from build123d import *

# Parameters (mm, degrees)
BOSS_EXTRUDE1_DEPTH = 20
BOSS_EXTRUDE2_DEPTH = 80
BOSS_EXTRUDE6_DEPTH = 30
BOSS_EXTRUDE7_DEPTH = 75
CUT_EXTRUDE1_REACH  = 158.605


with BuildPart() as part:
    # Sketch1 → Boss-Extrude1 (new body)
    with BuildSketch(Plane(origin=(0, 0, 0), x_dir=(1, 0, 0), z_dir=(0, 1, 0))):
        Polygon((35, 75), (0, 75), (0, 0), (65, 0), (65, 95), (35, 95), align=None)
    extrude(amount=BOSS_EXTRUDE1_DEPTH)

    # Sketch1<3> → Boss-Extrude2 (add)
    with BuildSketch(Plane(origin=(0, 0, 0), x_dir=(1, 0, 0), z_dir=(0, 1, 0))):
        Polygon((15, 130), (15, 100), (0, 100), (0, 75), (35, 75), (35, 95), (65, 95), (65, 100), (65, 130), align=None)
    extrude(amount=BOSS_EXTRUDE2_DEPTH)

    # Sketch8 → Boss-Extrude6 (add)
    with BuildSketch(Plane(origin=(65, 0, 0), x_dir=(0, 0, -1), z_dir=(1, 0, 0))):
        Polygon((95, 57.913643311), (50, 57.913643311), (0, 20), (95, 20), align=None)
    extrude(amount=-BOSS_EXTRUDE6_DEPTH)

    # Sketch9 → Boss-Extrude7 (add)
    with BuildSketch(Plane.XY.offset(-75)):
        Polygon((0, 20), (35, 57.913643311), (35, 20), align=None)
    extrude(amount=BOSS_EXTRUDE7_DEPTH)

    # Sketch10 → Cut-Extrude1 (cut, up to next)
    with BuildSketch(Plane(origin=(35, 0, 0), x_dir=(0, 0, -1), z_dir=(1, 0, 0)), mode=Mode.PRIVATE) as cut_extrude1_sk1:
        Polygon((0, 57.913643311), (50, 57.913643311), (0, 20), align=None)
    cut_extrude1_tool1 = extrude(cut_extrude1_sk1.sketch, amount=-CUT_EXTRUDE1_REACH, mode=Mode.PRIVATE) & part.part
    add(cut_extrude1_tool1.solids().sort_by_distance((35, 45.275762, -16.666667))[0], mode=Mode.SUBTRACT)


solid = part.part
Verification items for the finished model (mm, model axes). A direction names the side the tool comes from. Coordinates: 2 decimals unless noted, no trailing zeros. Loops run counter-clockwise (first coordinate to the right, second up) from the corner with the lowest first, then second, coordinate; pieces in that order, holes last. Notation, with made-up numbers: (-21, 65) -> (38, 65) arc R23 cw to (38, 92) -> close; hole circle Ø2 at (-39.5, 21). An arc over 180 degrees is marked (long way). Answer as CSV lines item,"result".
1) Thickness scan on L1, parallel to Y at x = 62, z = -56.5; L2, parallel to Z at x = 10.5, y = 8.5; L3, parallel to Z at x = 18.5, y = 54.5. Record the ranges inside material, lowest first. Write a range as from..to.
Found:
L1,"y = 0..57.91"
L2,"z = -100..0"
L3,"z = -130..-75"
2) Cross-section at D-D, the plane z = -66.5. Record the cut outline in (x, y).
Found:
outline,"(0, 0) -> (65, 0) -> (65, 57.91) -> (35, 57.91) -> (0, 20) -> close"
3) Tool access check on faces 1 (the flat face through (15, 39, -115)), 2 (the flat face through (13, 56, -75)), 3 (the flat face through (50, 69, -95)). Record the directions out of +Z, -Z, +X, -X, +Y, -Y that give a thin tool (end or side, any length) a straight path to the whole face; none if there is none.
Found:
face 1,"-Z, -X, +Y, -Y"
face 2,"+Z, -X, +Y"
face 3,"+Z, +X, +Y"
4) Cross-section at C-C, the plane y = 61. Record the cut outline in (x, z).
Found:
outline,"(0, -100) -> (15, -100) -> (15, -130) -> (65, -130) -> (65, -95) -> (35, -95) -> (35, -75) -> (0, -75) -> close"
5) Depth check by flat-ended pin: pin 1 (6 mm diameter, centred on x = 39, z = -30.5, fed in from +Y); pin 2 (10.5 mm diameter, centred on x = 14, y = 48, fed in from +Z); pin 3 (6 mm diameter, centred on y = 68.5, z = -85, fed in from +X). Enter the tip coordinate at first touch or a pass-through.
Found:
pin 1,"stops at y = 45.4"
pin 2,"stops at z = -75"
pin 3,"stops at x = 35"
6) Cross-section at B-B, the plane z = -92. Record the cut outline in (x, y), then the cut area to 3 significant figures.
Found:
outline,"(0, 0) -> (65, 0) -> (65, 57.91) -> (35, 57.91) -> (35, 80) -> (0, 80) -> close"
area,"4,540 mm2"
7) Cross-section at A-A, the plane x = 59. Record the cut outline in (y, z).
Found:
outline,"(0, -130) -> (80, -130) -> (80, -95) -> (57.91, -95) -> (57.91, -50) -> (20, 0) -> (0, 0) -> close"
